from build123d import *

# Parameters (mm, degrees)
SKETCH1_R           = 3
BOSS_EXTRUDE1_DEPTH = 1.5
SKETCH2_R           = 3
BOSS_EXTRUDE2_DEPTH = 12.7
SKETCH3_R           = 11.04
BOSS_EXTRUDE3_DEPTH = 1.524
FILLET1_R           = 7.62
SKETCH4_R           = 8.5
CUT_EXTRUDE1_DEPTH  = 13.724


with BuildPart() as part:
    # Sketch1 → Boss-Extrude1 (new body, symmetric)
    with BuildSketch(Plane.XY):
        with BuildLine():
            Line((-31.75, 5), (31.75, 5))
            ThreePointArc((31.75, 5), (36.75, 0), (31.75, -5))
            Line((31.75, -5), (-31.75, -5))
            ThreePointArc((-31.75, -5), (-36.75, 0), (-31.75, 5))
        make_face()
        with Locations((-31.75, 0)):
            Circle(SKETCH1_R, mode=Mode.SUBTRACT)
        with Locations((31.75, 0)):
            Circle(SKETCH1_R, mode=Mode.SUBTRACT)
    extrude(amount=BOSS_EXTRUDE1_DEPTH, both=True)

    # Sketch2 → Boss-Extrude2 (add)
    with BuildSketch(Plane.XY.offset(1.5)):
        with Locations((-31.75, 0)):
            Circle(SKETCH2_R)
    extrude(amount=-BOSS_EXTRUDE2_DEPTH)

    # Sketch3 → Boss-Extrude3 (add, symmetric)
    with BuildSketch(Plane.XY):
        with Locations((31.75, 0)):
            Circle(SKETCH3_R)
    extrude(amount=BOSS_EXTRUDE3_DEPTH, both=True)

    # Fillet1
    fillet1_edges = [part.edges().sort_by_distance(p)[0] for p in [
        (21.907154883, 5, 0),
        (21.907154883, -5, 0),
    ]]
    fillet(fillet1_edges, radius=FILLET1_R)

    # Sketch4 → Cut-Extrude1 (cut, through all)
    with BuildSketch(Plane.XY.offset(1.524)):
        with Locations((31.75, 0)):
            Circle(SKETCH4_R)
    extrude(amount=-CUT_EXTRUDE1_DEPTH, mode=Mode.SUBTRACT)


solid = part.part
The model under review builds one solid part; all positions refer to its coordinate system, in mm. A direction names the side the tool comes from. Give positions to 0.01 mm unless a question says otherwise; leave off trailing zeros. Order: outer loops, then holes, each group sorted by start corner. A loop starts at its lowest first (then second) coordinate and runs counter-clockwise, first axis right, second up. Notation, with made-up numbers: M 17,16.5 L 38,16.5 A21 cw 38,51.5 Z; hole C -38,38.5 d2. An arc over 180 degrees is marked long. Answer in a Markdown table with one row per item. Add a question column.
1. To check wall thickness, follow line 1 along Y through (x, z) = (31.75, 0.9); line 2 along X through (y, z) = (0.25, -9.5); line 3 along Z through (x, y) = (-31.5, 0). State the ranges of each line that lie inside material, in increasing order.
2. Machinability: for faces 1 (the flat face through (-7, -5, 0)), 2 (the flat face through (-32, 0, -11.2)), 3 (the flat face through (38, -6, -1.524)), which of the approach directions +Z, -Z, +X, -X, +Y, -Y give a long, thin tool a straight path to every point of the face, cutting with its end or side? Answer none if there is none.
3. Mouldability with a two-part tool opening along Y and no side actions: class faces 4 (the cylindrical face through (-34.747, 0.132, -6.282)), 5 (the flat face through (-7, 5, 0)), 6 (the cylindrical face through (36.32, 7.167, 0.021)), 7 (the flat face through (-6, 0, 1.5)) as released by +Y, released by -Y, zero draft, split by the parting line, or undercut.
4. Add section C-C on x = 13.5. State the section outline as (y, z) points.
5. Add section D-D on z = -8.5. State the section outline as (x, y) points, plus the area to 3 significant figures.
6. Add section A-A on x = 31.75. State the section outline as (y, z) points.
7. For pin 1 Ø10 at (x, y) = (-12.5, -5.5) entering from -Z; pin 2 Ø3.5 at (x, z) = (-14, 0) entering from +Y; pin 3 Ø0.9 at (x, z) = (4.5, -0.5) entering from -Y, all flat-tipped, find the tip position at first contact; note any pin that passes through.
The answers:
| question | item | result |
|---|---|---|
| 1 | line 1 | -11.04 to -8.5, 8.5 to 11.04 |
| 1 | line 2 | -34.74 to -28.76 |
| 1 | line 3 | -11.2 to 1.5 |
| 2 | face 1 | +Z, -Z, -X, -Y |
| 2 | face 2 | -Z, +X, -X, +Y, -Y |
| 2 | face 3 | -Z, +X, +Y, -Y |
| 3 | face 4 | split by the parting line |
| 3 | face 5 | released by +Y |
| 3 | face 6 | undercut |
| 3 | face 7 | zero draft |
| 4 | outline | M -5,-1.5 L 5,-1.5 L 5,1.5 L -5,1.5 Z |
| 5 | outline | C -31.75,0 d6 |
| 5 | area | 28.3 mm2 |
| 6 | outline | M -11.04,-1.52 L -8.5,-1.52 L -8.5,1.52 L -11.04,1.52 Z; M 8.5,-1.52 L 11.04,-1.52 L 11.04,1.52 L 8.5,1.52 Z |
| 7 | pin 1 | z = -1.5 |
| 7 | pin 2 | y = 5 |
| 7 | pin 3 | y = -5 |
